Check sheet for the modelled part. Datum: model origin and axes. Units: mm. A direction names the side the tool comes from. Round coordinates to 2 decimals unless told otherwise and drop trailing zeros. Loops run counter-clockwise (first coordinate to the right, second up) from the corner with the lowest first, then second, coordinate; pieces in that order, holes last. Notation, with made-up numbers: (37.25, -19.75) -> (48.25, -19.75) arc R38 cw to (48.25, 19.25) -> close; hole circle Ø11 at (74, 52.25). An arc over 180 degrees is marked (long way). One line per item, written item: value. Start each with the question number.
1. Release check for a two-part mould opening along Y. For faces 3 (the face through (-182.12, -5.17, 28.67)), 4 (the face through (-36.74, -4.7, 36.46)), 5 (the face through (-100, -9.525, 29)) record: +Y half, -Y half, draft (parallel to the pull), parting line (faces both ways), or undercut.
2. Cross-section at B-B on z = 22.5. Count the separate pieces of the cut face and the enclosed holes in it, then the cut area to 3 significant figures.
3. Set-up check for faces 1 (the face through (-36.83, -4.7, 21.13)), 2 (the face through (-20.636, -4.832, 28.573)): record each of +Z, -Z, +X, -X, +Y, -Y from which the full face is reachable in a straight line by a thin tool's end or side.
4. Material ranges on L1, parallel to X at y = -9, z = 41.5; L2, parallel to Z at x = -190.5, y = -5; L3, parallel to X at y = -8.5, z = 29.5 (3 decimals), recorded low to high.
5. Go/stop test with flat-tipped pins: pin 1 (5 mm diameter, centred on y = -6.5, z = 42.5, fed in from -X); pin 2 (2.5 mm diameter, centred on x = -177.8, y = -4.76, fed in from +Z); pin 3 (4.5 mm diameter, centred on y = -4.76, z = 28.84, fed in from +X). Record where each tip stops, or that it passes through.
6. Cross-section at A-A on x = -69. Record the cut outline in (y, z) (3 decimals).
from build123d import *

# Parameters (mm, degrees)
F0_W      = 196.85
F0_H      = 38.1
F1_DEPTH  = 9.525
F2_R      = 6.35
F3_R      = 6.35
F4_W      = 50.8
F4_H      = 19.05
F5_DEPTH  = 25.4
F6_R      = 6.35
F7_R      = 6.35
F8_R      = 6.35
F9_R      = 6.35
F10_W     = 50.8
F10_H     = 19.05
F11_DEPTH = 25.4
F12_R     = 6.35
F13_R     = 5.08
F14_R     = 6.35
F15_R     = 6.35
F16_R     = 1.905
F18_DEPTH = 25.4
F20_R     = 1.5875
F21_DEPTH = 48.006
F22_R     = 1.5875
F23_DEPTH = 44.3738
F26_D     = 3.81
F27_D     = 5.1054
F27_DEPTH = 13.462
F27_TIP   = 1.5338169022
F28_D     = 5.1054
F28_DEPTH = 13.462
F28_TIP   = 1.5338169022
F29_R     = 6.35


with BuildPart() as f1:
    # F0 (on Front) → F1 (new body)
    with BuildSketch(Plane.XZ):
        with Locations((-98.425, 28.8397434607)):
            Rectangle(F0_W, F0_H)
    extrude(amount=F1_DEPTH)

    # F2
    f2_edges = [f1.edges().sort_by_distance(p)[0] for p in [
        (0, -4.7625, 9.789743),
    ]]
    fillet(f2_edges, radius=F2_R)

    # F3
    f3_edges = [f1.edges().sort_by_distance(p)[0] for p in [
        (-196.85, -4.7625, 9.789743),
    ]]
    fillet(f3_edges, radius=F3_R)

    # F4 (on face) → F5 (cut)
    with BuildSketch(Plane.XZ.offset(9.525)):
        with Locations((-136.525, 28.8397434607)):
            Rectangle(F4_W, F4_H)
    extrude(amount=-F5_DEPTH, mode=Mode.SUBTRACT)

    # F6
    f6_edges = [f1.edges().sort_by_distance(p)[0] for p in [
        (-161.925, -4.7625, 38.364743),
    ]]
    fillet(f6_edges, radius=F6_R)

    # F7
    f7_edges = [f1.edges().sort_by_distance(p)[0] for p in [
        (-161.925, -4.7625, 19.314743),
    ]]
    fillet(f7_edges, radius=F7_R)

    # F8
    f8_edges = [f1.edges().sort_by_distance(p)[0] for p in [
        (-111.125, -4.7625, 19.314743),
    ]]
    fillet(f8_edges, radius=F8_R)

    # F9
    f9_edges = [f1.edges().sort_by_distance(p)[0] for p in [
        (-111.125, -4.7625, 38.364743),
    ]]
    fillet(f9_edges, radius=F9_R)

    # F10 (on face) → F11 (cut)
    with BuildSketch(Plane.XZ.offset(9.525)):
        with Locations((-60.325, 28.8397434607)):
            Rectangle(F10_W, F10_H)
    extrude(amount=-F11_DEPTH, mode=Mode.SUBTRACT)

    # F12
    f12_edges = [f1.edges().sort_by_distance(p)[0] for p in [
        (-85.725, -4.7625, 38.364743),
    ]]
    fillet(f12_edges, radius=F12_R)

    # F13
    f13_edges = [f1.edges().sort_by_distance(p)[0] for p in [
        (-85.725, -4.7625, 19.314743),
    ]]
    fillet(f13_edges, radius=F13_R)

    # F14
    f14_edges = [f1.edges().sort_by_distance(p)[0] for p in [
        (-34.925, -4.7625, 19.314743),
    ]]
    fillet(f14_edges, radius=F14_R)

    # F15
    f15_edges = [f1.edges().sort_by_distance(p)[0] for p in [
        (-34.925, -4.7625, 38.364743),
    ]]
    fillet(f15_edges, radius=F15_R)

    # F16 (on face) → F18 (cut)
    with BuildSketch(Plane.XZ.offset(9.525)):
        with Locations((-190.5, 41.5397434607)):
            Circle(F16_R)
        with Locations((-161.925, 41.5397434607)):
            Circle(F16_R)
        with Locations((-161.925, 16.1594711244)):
            Circle(F16_R)
        with Locations((-190.5, 16.1397434607)):
            Circle(F16_R)
    extrude(amount=-F18_DEPTH, mode=Mode.SUBTRACT)

    # F20 (on face) → F21 (cut)
    with BuildSketch(Plane(origin=(0, 0, 9.7897434607), x_dir=(1, 0, 0), z_dir=(0, 0, -1))):
        with Locations((-177.8, 4.7625)):
            Circle(F20_R)
    extrude(amount=-F21_DEPTH, mode=Mode.SUBTRACT)

    # F22 (on face) → F23 (cut)
    with BuildSketch(Plane(origin=(0, 0, 9.7897434607), x_dir=(1, 0, 0), z_dir=(0, 0, -1))):
        with Locations((-19.05, 4.7625)):
            Circle(F22_R)
    extrude(amount=-F23_DEPTH, mode=Mode.SUBTRACT)

    # F26 (through all)
    with Locations(Plane(origin=(0, 0, 9.7897434607), x_dir=(1, 0, 0), z_dir=(0, 0, -1))):
        with Locations((-60.325, 4.7625), (-136.525, 4.7625)):
            Hole(F26_D / 2)

    # F27
    with Locations(Plane.YZ):
        with Locations((-4.7625, 28.8397434607)):
            Hole(F27_D / 2, depth=F27_DEPTH)
            with Locations((0, 0, -(F27_DEPTH + F27_TIP / 2))):  # 118° drill point
                Cone(0, F27_D / 2, F27_TIP, mode=Mode.SUBTRACT)

    # F28
    with Locations(Plane(origin=(-196.85, 0, 0), x_dir=(0, -1, 0), z_dir=(-1, 0, 0))):
        with Locations((4.7625, 28.8397434607)):
            Hole(F28_D / 2, depth=F28_DEPTH)
            with Locations((0, 0, -(F28_DEPTH + F28_TIP / 2))):  # 118° drill point
                Cone(0, F28_D / 2, F28_TIP, mode=Mode.SUBTRACT)

    # F29
    f29_edges = [f1.edges().sort_by_distance(p)[0] for p in [
        (-196.85, -4.7625, 47.889743),
        (0, -4.7625, 47.889743),
    ]]
    fillet(f29_edges, radius=F29_R)


solid = f1.part
Taken from the geometry:
1. face 3: undercut
1. face 4: draft
1. face 5: -Y half
2. separate pieces: 3
2. enclosed holes: 2
2. area: 919 mm2
3. face 1: +Y, -Y
3. face 2: +Z, -Z
4. L1: x = -196.85 to -192.4, -188.6 to -163.83, -160.02 to 0
4. L2: z = 9.79 to 14.23, 18.04 to 26.3, 31.38 to 39.63, 43.44 to 47.89
4. L3: x = -196.85 to -161.925, -111.125 to -85.725, -34.925 to 0
5. pin 1: stops at x = -196.85
5. pin 2: passes through
5. pin 3: stops at x = -13.64
6. outline: (-9.525, 9.79) -> (0, 9.79) -> (0, 19.315) -> (-9.525, 19.315) -> close; (-9.525, 38.365) -> (0, 38.365) -> (0, 47.89) -> (-9.525, 47.89) -> close
